from build123d import *

# Parameters (mm, degrees)
F0_R     = 46.99
F2_R     = 46.99
F4_T     = -2.54
F6_R     = 50.8
F6_R_2   = 44.45
F7_DEPTH = 2.54


with BuildPart() as f3:
    # F0 (on Top) → F3 section 0
    with BuildSketch(Plane.XY):
        Circle(F0_R)
    # F2 (on offset) → F3 section 1
    with BuildSketch(Plane.XY.offset(76.2)):
        Circle(F2_R)
    loft()

    # F4
    f4_openings = [f3.faces().sort_by_distance(p)[0] for p in [
        (0, 0, 76.2),
    ]]
    offset(amount=F4_T, openings=f4_openings)

    # F6 (on offset) → F7 (join)
    with BuildSketch(Plane.XY.offset(78.74)):
        Circle(F6_R)
        Circle(F6_R_2, mode=Mode.SUBTRACT)
    extrude(amount=-F7_DEPTH)


solid = f3.part
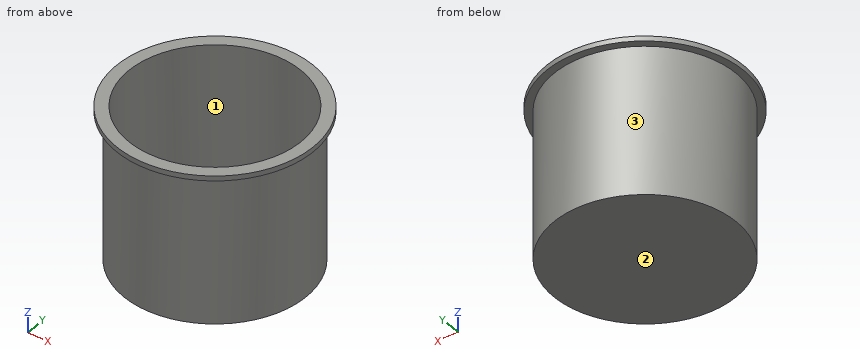
Input: part model. Units: mm. Frame: model coordinates. Face numbers are marked on the shaded views. Give positions to 0.01 mm unless a question says otherwise; leave off trailing zeros. Write each loop counter-clockwise with the first axis right and the second up, starting at its lowest first coordinate (ties: lowest second). Pieces come first, ordered by that corner, then holes. Notation, with made-up numbers: M -36.75,-28 L -29.75,-28 A19 ccw -29.75,4 Z; hole C 55.5,77.5 d9. An arc over 180 degrees is marked long. Write item = value, one per line. Start each with the question number.
1) Cut plane A-A on x = 0. Return the cut outline in (y, z), then the cut area to 3 significant figures.
2) First-contact query: pin 1 Ø12 at (y, z) = (40.5, 46) entering from -X; pin 2 Ø4 at (x, z) = (37, 37) entering from -Y; pin 3 Ø1.5 at (x, z) = (31, 65.5) entering from -Y. Flat tips, straight axial feed; report the tip coordinate or a pass-through.
3) Material intervals for line 1 along Y through (x, z) = (0, 36); line 2 along Z through (x, y) = (-39, -13); line 3 along X through (y, z) = (-31, 12), sorted ascending. Write a range as [from, to].
4) Cut plane B-B on y = 4.5. Return the cut outline in (x, z), then the cut area to 3 significant figures.
5) Draft query along Y for the marked faces 1, 2 and 3. Return one class per face: +Y half, -Y half, draft (parallel to the pull), parting line (faces both ways), or undercut.
6) Cut plane C-C on z = 37. Return the cut outline in (x, y), then the cut area to 3 significant figures.
Solved:
q1.outline = M -50.8,76.2 L -46.99,76.2 L -46.99,0 L 46.99,0 L 46.99,76.2 L 50.8,76.2 L 50.8,78.74 L 44.45,78.74 L 44.45,2.54 L -44.45,2.54 L -44.45,78.74 L -50.8,78.74 Z
q1.area = 645 mm2
q2.pin_1 = -31.9
q2.pin_2 = -31.35
q2.pin_3 = -35.96
q3.line_1 = [-46.99, -44.45], [44.45, 46.99]
q3.line_2 = [0, 2.54]
q3.line_3 = [-35.31, -31.86], [31.86, 35.31]
q4.outline = M -50.6,76.2 L -46.77,76.2 L -46.77,0 L 46.77,0 L 46.77,76.2 L 50.6,76.2 L 50.6,78.74 L 44.22,78.74 L 44.22,2.54 L -44.22,2.54 L -44.22,78.74 L -50.6,78.74 Z
q4.area = 646 mm2
q5.face_1 = undercut
q5.face_2 = draft
q5.face_3 = parting line
q6.outline = C 0,0 d93.98; hole C 0,0 d88.9
q6.area = 730 mm2
